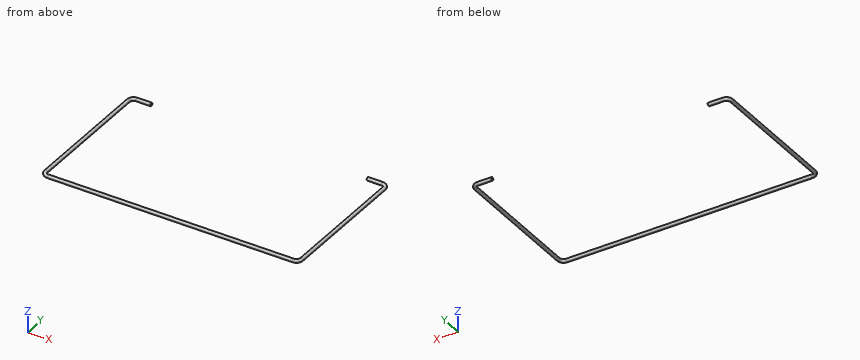
from build123d import *

# Parameters (mm, degrees)
F1_R = 2.5


with BuildPart() as f2:
    # F2: sweep along a path in F0
    with BuildLine(Plane.XY) as f2_path:
        Line((0, 0), (-22, 0))
        ThreePointArc((-22, 0), (-27.6568542495, -2.3431457505), (-30, -8))
        Line((-30, -8), (-30, -207))
        ThreePointArc((-30, -207), (-27.6568542495, -212.6568542495), (-22, -215))
        Line((-22, -215), (352, -215))
        ThreePointArc((352, -215), (357.6568542495, -212.6568542495), (360, -207))
        Line((360, -207), (360, -8))
        ThreePointArc((360, -8), (357.6568542495, -2.3431457505), (352, 0))
        Line((352, 0), (330, 0))
    # F1 (on Right) → F2 (sweep)
    with BuildSketch(Plane.YZ):
        Circle(F1_R)
    sweep(path=f2_path.line)


solid = f2.part
Check sheet for the modelled part. Datum: model origin and axes. Units: mm. Give positions to 0.01 mm unless a question says otherwise; leave off trailing zeros. Loops run counter-clockwise (first coordinate to the right, second up) from the corner with the lowest first, then second, coordinate; pieces in that order, holes last. Notation, with made-up numbers: M 38.5,31 L 63.5,31 A20 cw 63.5,48 Z; hole C 66.25,89 d10. An arc over 180 degrees is marked long. Return JSON: item names as keys, results as strings. Group by question number.
1. Cross-section at C-C on x = 273. Record the boundary of the cut face in (y, z).
2. Thickness scan on L1, parallel to Y at x = -2, z = 0.4; L2, parallel to Y at x = -17, z = 0.5; L3, parallel to X at y = -135.5, z = 0.2. Record the ranges inside material, lowest first.
3. Go/stop test with flat-tipped pins: pin 1 (1.5 mm diameter, centred on y = 1, z = -0.5, fed in from +X); pin 2 (1.5 mm diameter, centred on y = -1, z = -1, fed in from -X). Record where each tip stops, or that it passes through.
4. Cross-section at B-B on z = 1.5. Record the boundary of the cut face in (x, y).
5. Cross-section at A-A on y = -125. Record the boundary of the cut face in (x, z).
Return value:
{
 "1": {"outline": "C -215,0 d5"},
 "2": {"L1": "-217.47 to -212.53, -2.47 to 2.47", "L2": "-217.45 to -212.55, -2.45 to 2.45", "L3": "-32.49 to -27.51, 357.51 to 362.49"},
 "3": {"pin 1": "x = 358.44", "pin 2": "x = -30.27"},
 "4": {"outline": "M -32,-207 A10 ccw -22,-217 L 352,-217 A10 ccw 362,-207 L 362,-8 A10 ccw 352,2 L 330,2 L 330,-2 L 352,-2 A6 cw 358,-8 L 358,-207 A6 cw 352,-213 L -22,-213 A6 cw -28,-207 L -28,-8 A6 cw -22,-2 L 0,-2 L 0,2 L -22,2 A10 ccw -32,-8 Z"},
 "5": {"outline": "C -30,0 d5; C 360,0 d5"}
}
